Input: part model. Units: mm. Frame: model coordinates. Coordinates: 2 decimals unless noted, no trailing zeros. Loops run counter-clockwise (first coordinate to the right, second up) from the corner with the lowest first, then second, coordinate; pieces in that order, holes last.
```python
from build123d import *

# Parameters (mm, degrees)
SKETCH2_W                   = 101.6
SKETCH2_H                   = 78.74
SQUARE_DEPTH                = 5.334
SKETCH4_R                   = 2.975000019
SKETCH4_W                   = 19.05
SKETCH4_H                   = 5.334
MOUNTING_POINTS_DEPTH       = 65.490995154
TRICUT_DEPTH                = 65.490995154
TRICUT_DEPTH_BACK           = 65.490995154
SKETCH5_W                   = 19.05
SKETCH5_H                   = 5.334
BOTTOMTEETH_DEPTH           = 5.334
SKETCH8_W                   = 5.334
SKETCH8_H                   = 19.05
GRABBERSTOP_DEPTH           = 10.4
UNOPLATFORM_DEPTH           = 5.334
SKETCH13_W                  = 19.05
SKETCH13_H                  = 5.334
BACKTOOTH_DEPTH             = 5.334
SKETCH14_W                  = 5.334
SKETCH14_H                  = 24.923365698
CIRCUITSTACKEXTENSION_DEPTH = 25.4
SKETCH16_W                  = 5.334
SKETCH16_H                  = 15.24
CIRCUITSTACKHOLDER_DEPTH    = 131.051294604
SKETCH17_W                  = 16.51
SKETCH17_H                  = 5.334
BRACES_DEPTH                = 63.5
SKETCH18_W                  = 5.334
SKETCH18_H                  = 12.7
BRACE2_DEPTH                = 12.7
SKETCH19_W                  = 7.366
SKETCH19_H                  = 5.334
BRACE3_DEPTH                = 12.7
SKETCH20_W                  = 12.499999892
SKETCH20_H                  = 18.7
ON_OFF_SWITCH_DEPTH         = 132.609742414


with BuildPart() as part:
    # Sketch2 → square (new body)
    with BuildSketch(Plane.XY):
        Rectangle(SKETCH2_W, SKETCH2_H)
    extrude(amount=SQUARE_DEPTH)

    # Sketch4 → Mounting points (cut, through all)
    with BuildSketch(Plane.XY.offset(5.334)):
        with Locations((38.1, 31.496)):
            Circle(SKETCH4_R)
        with Locations((24.040000053, -17.113634263)):
            Rectangle(SKETCH4_W, SKETCH4_H)
    extrude(amount=-MOUNTING_POINTS_DEPTH, mode=Mode.SUBTRACT)

    # Sketch3 → tricut (cut, two sides: drawn at the far end of the back side and taken through both)
    with BuildSketch(Plane.XY.offset(5.334).offset(-TRICUT_DEPTH_BACK)):
        Polygon((-207.681606875, -255.517991695), (-50.8, -39.37), (6.35, 39.37), (50.8, 39.37), (317.880124475, 39.37), (56.500793408, 505.211192735), (-469.060937942, 210.323201041), align=None)
    extrude(amount=TRICUT_DEPTH + TRICUT_DEPTH_BACK, mode=Mode.SUBTRACT)

    # Sketch5 → bottomTeeth (add)
    with BuildSketch(Plane.XZ.offset(39.37)):
        with Locations((-41.275, 2.667)):
            Rectangle(SKETCH5_W, SKETCH5_H)
        with Locations((0, 2.667)):
            Rectangle(SKETCH5_W, SKETCH5_H)
        with Locations((41.275, 2.667)):
            Rectangle(SKETCH5_W, SKETCH5_H)
    extrude(amount=BOTTOMTEETH_DEPTH)

    # Sketch8 → GrabberStop (add)
    with BuildSketch(Plane(origin=(50.8, 0, 0), x_dir=(0, 0, -1), z_dir=(1, 0, 0))):
        with Locations((-2.667, 23.495)):
            Rectangle(SKETCH8_W, SKETCH8_H)
    extrude(amount=GRABBERSTOP_DEPTH)

    # Sketch9 → UnoPlatform (add)
    with BuildSketch(Plane.XY.offset(5.334)):
        Polygon((-96.60999982, -39.37), (-50.8, -39.37), (-32.71046038, -14.446634302), (-96.60999982, -14.446634302), align=None)
    extrude(amount=-UNOPLATFORM_DEPTH)

    # Sketch13 → backTooth (cut)
    with BuildSketch(Plane(origin=(0, -14.446634302, 0), x_dir=(1, 0, 0), z_dir=(0, 1, 0))):
        with Locations((-74.38499982, -2.667)):
            Rectangle(SKETCH13_W, SKETCH13_H)
    extrude(amount=-BACKTOOTH_DEPTH, mode=Mode.SUBTRACT)

    # Sketch14 → CircuitStackExtension (add)
    with BuildSketch(Plane.ZY.offset(96.60999982)):
        with Locations((2.667, -26.908317151)):
            Rectangle(SKETCH14_W, SKETCH14_H)
    extrude(amount=CIRCUITSTACKEXTENSION_DEPTH)

    # Sketch16 → CircuitStackHolder (cut, through all)
    with BuildSketch(Plane.XY.offset(5.334)):
        with Locations((-103.08699982, -22.066634302)):
            Rectangle(SKETCH16_W, SKETCH16_H)
    extrude(amount=-CIRCUITSTACKHOLDER_DEPTH, mode=Mode.SUBTRACT)

    # Sketch17 → Braces (add)
    with BuildSketch(Plane(origin=(0, -14.446634302, 0), x_dir=(1, 0, 0), z_dir=(0, 1, 0))):
        with Locations((-92.16499982, -2.667)):
            Rectangle(SKETCH17_W, SKETCH17_H)
    extrude(amount=BRACES_DEPTH)

    # Sketch18 → Brace2 (add)
    with BuildSketch(Plane.ZY.offset(100.41999982)):
        with Locations((2.667, 30.003365698)):
            Rectangle(SKETCH18_W, SKETCH18_H)
    extrude(amount=BRACE2_DEPTH)

    # Sketch19 → Brace3 (add)
    with BuildSketch(Plane(origin=(0, 36.353365698, 0), x_dir=(1, 0, 0), z_dir=(0, 1, 0))):
        with Locations((-109.43699982, -2.667)):
            Rectangle(SKETCH19_W, SKETCH19_H)
    extrude(amount=BRACE3_DEPTH)

    # Sketch20 → On_Off Switch (cut, through all)
    with BuildSketch(Plane.XY.offset(5.334)):
        with Locations((0.100000054, 1.73)):
            Rectangle(SKETCH20_W, SKETCH20_H)
    extrude(amount=-ON_OFF_SWITCH_DEPTH, mode=Mode.SUBTRACT)


solid = part.part
```
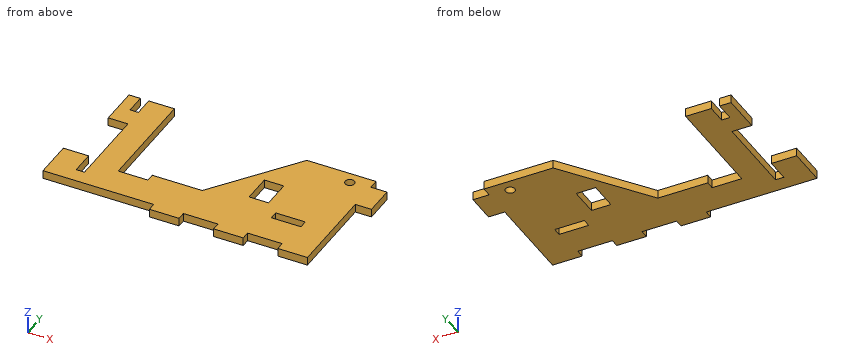
Item 1: Section query A-A (x = 25). Output: boundary loops of the cut face in (y, z), then the cut area to 3 significant figures.
Result:
outline: (-39.37, 0) - (-19.78, 0) - (-19.78, 5.33) - (-39.37, 5.33) - close; (-14.45, 0) - (39.37, 0) - (39.37, 5.33) - (-14.45, 5.33) - close
area: 392 mm2
Item 2: Section query D-D (x = -104). Output: boundary loops of the cut face in (y, z).
Result:
outline: (-39.37, 0) - (-29.69, 0) - (-29.69, 5.33) - (-39.37, 5.33) - close; (23.65, 0) - (36.35, 0) - (36.35, 5.33) - (23.65, 5.33) - close
Item 3: Section query B-B (y = -17). Output: boundary loops of the cut face in (x, z) (3 decimals).
Result:
outline: (-122.01, 0) - (-105.754, 0) - (-105.754, 5.334) - (-122.01, 5.334) - close; (-100.42, 0) - (-83.91, 0) - (-83.91, 5.334) - (-100.42, 5.334) - close; (-64.86, 0) - (14.515, 0) - (14.515, 5.334) - (-64.86, 5.334) - close; (33.565, 0) - (50.8, 0) - (50.8, 5.334) - (33.565, 5.334) - close
Item 4: Contact query for flat-ended pins moving along their axis: P1, Ø2.5, axis at y = -43, z = 3, coming from the +X side; P2, Ø1.6, axis at y = -4.5, z = 4, coming from the -X side; P3, Ø1.6, axis at x = 3, z = 4, coming from the +Y side. Output: stop coordinate, or through.
Result:
P1: stops at x = 50.8
P2: stops at x = -100.42
P3: stops at y = 35.86
Item 5: Section query C-C (y = -0.5). Output: boundary loops of the cut face in (x, z).
Result:
outline: (-100.42, 0) - (-83.91, 0) - (-83.91, 5.33) - (-100.42, 5.33) - close; (-22.59, 0) - (-6.15, 0) - (-6.15, 5.33) - (-22.59, 5.33) - close; (6.35, 0) - (50.8, 0) - (50.8, 5.33) - (6.35, 5.33) - close
Item 6: Line query: L1, parallel to X at y = -15, z = 4.4 (3 decimals); L2, parallel to Y at x = 38.1, z = 3.1; L3, parallel to Y at x = 22, z = 0.95. Output: solid intervals per line, ascending.
Result:
L1: x = -122.01 to -105.754, -100.42 to -83.91, -64.86 to 14.515, 33.565 to 50.8
L2: y = -44.7 to 28.52, 34.47 to 39.37
L3: y = -39.37 to -19.78, -14.45 to 39.37
